Could you check a few things on this model? Use its own coordinates, in mm. A direction names the side the tool comes from. Round coordinates to 2 decimals unless told otherwise and drop trailing zeros. Write each loop counter-clockwise with the first axis right and the second up, starting at its lowest first coordinate (ties: lowest second). Pieces come first, ordered by that corner, then holes. Notation, with made-up numbers: (3, 59.25) -> (40, 59.25) arc R8 cw to (40, 70.25) -> close; hole circle Ø8 at (44, 66.5). An arc over 180 degrees is marked (long way). Answer in a Markdown table with one row per item. Add a question column.
Autodesk Inventor part; units mm, degrees
ref_plane "YZ Plane" through (0, 0, 0) normal (1, 0, 0) x (0, 1, 0)
ref_plane "XZ Plane" through (0, 0, 0) normal (0, 1, 0) x (-1, 0, 0)
ref_plane "XY Plane" through (0, 0, 0) normal (0, 0, 1) x (1, 0, 0)
sketch "草图2" plane through (0, 0, 0) normal (0, 1, 0) x (-1, 0, 0)
  line L0 (-21, 21) -> (21, 21)
  line L1 (21, 21) -> (21, -21)
  line L2 (21, -21) -> (-21, -21)
  line L3 (-21, -21) -> (-21, 21)
  line L4 (-21, 21) -> (21, -21) construction
  line L5 (21, 21) -> (-21, -21) construction
  point P0 (0, 0)
  dimension "d3" = 42
  dimension "d4" = 42
extrude "拉伸2" add sketch "草图2" along normal blind 3
sketch "草图3" plane through (-21, 0, 21) normal (0, 0, 1) x (1, 0, 0)
  line L0 (0, 3) -> (42, 3)
  line L1 (0, 3) -> (42, 3)
  line L2 (42, 3) -> (42, -40)
  line L3 (42, -40) -> (0, -40)
  line L4 (0, -40) -> (0, 3)
  point P0 (21, 0)
  dimension "d7" = 43
extrude "拉伸3" add sketch "草图3" along normal blind 3
sketch "草图7" plane through (0, 0, 0) normal (0, -1, 0) x (1, 0, 0)
  circle A0 centre (0, 0) radius 11.5
  circle A1 centre (-15.5, 15.5) radius 1.75
  circle A2 centre (-15.5, -15.5) radius 1.75
  circle A3 centre (15.5, -15.5) radius 1.75
  circle A4 centre (15.5, 15.5) radius 1.75
  dimension "d17" = 23
  dimension "d18" = 3.5
  dimension "d19" = 15.5
  dimension "d20" = 15.5
  dimension "d21" = 15.5
  dimension "d22" = 15.5
extrude "拉伸6" cut sketch "草图7" against normal blind 3
sketch "草图9" plane through (-21, 0, 21) normal (0, 0, -1) x (-1, 0, 0)
  circle A0 centre (-40, -6) radius 1.75
  line L0 (0, 0) -> (-42, 0)
  line L1 (-42, 3) -> (0, 3)
  line L2 (-21, 0) -> (-21, -40) construction
  line L3 (0, -40) -> (-42, -40)
  circle A1 centre (-2, -6) radius 1.75
  circle A2 centre (-32, -28) radius 1.75
  circle A3 centre (-10, -28) radius 1.75
  dimension "d32" = 3.5
  dimension "d34" = 9
  dimension "d35" = 19
  dimension "d36" = 3.5
  dimension "d37" = 11
  dimension "d38" = 22
extrude "拉伸8" cut sketch "草图9" against normal blind 10
sketch "草图10" plane through (21, 0, -21) normal (1, 0, 0) x (0, 0, -1)
  line L0 (0, 0) -> (-42, 0)
  line L1 (0, 0) -> (0, 3)
  line L2 (0, 3) -> (-45, 3)
  line L3 (-45, -40) -> (-45, 3)
  line L4 (-42, -40) -> (-45, -40)
  line L5 (-42, -40) -> (-42, 0)
  point P0 (-21, 0)
extrude "拉伸9" add sketch "草图10" along normal blind 2
sketch "草图11" plane through (-21, 0, -21) normal (-1, 0, 0) x (0, 0, 1)
  line L0 (42, 0) -> (0, 0)
  line L1 (42, 0) -> (42, -40)
  line L2 (42, -40) -> (45, -40)
  line L3 (45, 3) -> (45, -40)
  line L4 (0, 3) -> (45, 3)
  line L5 (0, 0) -> (0, 3)
  point P0 (21, 0)
extrude "拉伸10" add sketch "草图11" along normal blind 2
sketch "草图12" plane through (-21, 0, 24) normal (0, 0, 1) x (1, 0, 0)
  circle A0 centre (32, -28) radius 1.75
  circle A1 centre (40, -6) radius 1.75
  circle A2 centre (2, -6) radius 1.75
  circle A3 centre (10, -28) radius 1.75
  line L0 (44, -40) -> (-2, -40)
  line L1 (44, 3) -> (44, -40)
  line L2 (-2, 3) -> (44, 3)
  line L3 (-2, -40) -> (-2, 3)
  point P0 (21, 0)
extrude "拉伸11" add sketch "草图12" along normal blind 10
sketch "草图13" plane through (-21, 0, 21) normal (0, 0, -1) x (-1, 0, 0)
  circle A0 centre (-32, -28) radius 1.75
  circle A1 centre (-40, -6) radius 1.75
  circle A2 centre (-2, -6) radius 1.75
  circle A3 centre (-10, -28) radius 1.75
  line L0 (-44, 0) -> (2, 0)
  line L1 (-44, -40) -> (-44, 0)
  line L2 (-44, -40) -> (2, -40)
  line L3 (2, 0) -> (2, -40)
  point P0 (-21, 0)
extrude "拉伸12" cut sketch "草图13" against normal blind 10
properties part number "电机座2"
(1) Suppose I cut it at C-C, the plane y = -6. Please give me the cut outline in (x, z), then the cut area to 3 significant figures.
(2) Suppose I cut it at A-A, the plane x = 15.5. Please give me the cut outline in (y, z).
(3) On a 3-axis mill with a long thin cutter (end or side, diameter ignored), from which of +Z, -Z, +X, -X, +Y, -Y can I reach the whole of each face in a straight line? I mean faces 1 (the face through (5, 0, 11)), 2 (the face through (-9.331, -28.526, 32.479)). Say none if no direction works.
(4) I need wall thicknesses on L1, parallel to Z at x = 15.5, y = 0.7; L2, parallel to Z at x = 0, y = 0.8; L3, parallel to Y at x = 3.5, z = 27. Which ranges of each line are inside material? Lowest first, please.
(5) Suppose I cut it at B-B, the plane z = 0. Please give me the cut outline in (x, y), then the cut area to 3 significant figures.
(6) Suppose I cut it at D-D, the plane x = 0. Please give me the cut outline in (y, z), then the cut area to 3 significant figures.
(7) For P1, Ø4, axis at x = 11, y = -28, coming from the -Z side; P2, Ø3, axis at x = 15.5, z = -15.5, coming from the +Y side; P3, Ø2, axis at x = 17.5, z = 23.5, coming from the -Y side, each with a flat end and sliding along its axis, tell me the tip position at first contact or that it passes through.
(8) If we mould it in two halves opening along Z, with no side actions, what happens to faces 3 (the face through (0, -40, 32)), 4 (the face through (-14.6, 1.5, -14)), 5 (the face through (0, 1, -21)), 6 (the face through (-14.6, 1.5, 17))? For each: pulls with the +Z half, pulls with the -Z half, needs draft (parallel to the pull), parting line crosses it, or undercut.
Response:
| question | item | result |
|---|---|---|
| 1 | outline | (-23, 31) -> (-20.75, 31) -> (-20.75, 34) -> (-23, 34) -> close; (-17.25, 31) -> (17.25, 31) -> (17.25, 34) -> (-17.25, 34) -> close; (20.75, 31) -> (23, 31) -> (23, 34) -> (20.75, 34) -> close |
| 1 | area | 117 mm² |
| 2 | outline | (-40, 31) -> (0, 31) -> (0, 17.25) -> (3, 17.25) -> (3, 34) -> (-40, 34) -> close; (0, -21) -> (3, -21) -> (3, -17.25) -> (0, -17.25) -> close; (0, -13.75) -> (3, -13.75) -> (3, 13.75) -> (0, 13.75) -> close |
| 3 | face 1 | -Z, +X, -X, -Y |
| 3 | face 2 | +Z, -Z |
| 4 | L1 | -21 to -17.25, -13.75 to 13.75, 17.25 to 34 |
| 4 | L2 | -21 to -11.5, 11.5 to 34 |
| 4 | L3 | 0 to 3 |
| 5 | outline | (-23, 0) -> (-11.5, 0) -> (-11.5, 3) -> (-23, 3) -> close; (11.5, 0) -> (23, 0) -> (23, 3) -> (11.5, 3) -> close |
| 5 | area | 69.0 mm² |
| 6 | outline | (-40, 31) -> (0, 31) -> (0, 11.5) -> (3, 11.5) -> (3, 34) -> (-40, 34) -> close; (0, -21) -> (3, -21) -> (3, -11.5) -> (0, -11.5) -> close |
| 6 | area | 216 mm² |
| 7 | P1 | z = 31 |
| 7 | P2 | through |
| 7 | P3 | y = 0 |
| 8 | face 3 | needs draft |
| 8 | face 4 | undercut |
| 8 | face 5 | pulls with the -Z half |
| 8 | face 6 | undercut |
